Build history of the part. All positions in model axes, mm. Face numbers are marked on the shaded views. A direction names the side the tool comes from. Give positions to 0.01 mm unless a question says otherwise; leave off trailing zeros. Loops run counter-clockwise (first coordinate to the right, second up) from the corner with the lowest first, then second, coordinate; pieces in that order, holes last. Notation, with made-up numbers: M 38,-16 L 83,-16 A18 ccw 83,7 Z; hole C 20,70 d1. An arc over 180 degrees is marked long. Answer as a JSON object with one key per item and string values. Group by question number.
1. Slice it at A-A (y = 13.5). List the corners of the cut face in (x, z).
2. Slice it at B-B (z = 9.5). List the corners of the cut face in (x, y), then the cut area to 3 significant figures.
3. Slice it at C-C (x = -11.5). List the corners of the cut face in (y, z).
4. Mould opens along X. For the marked faces 3, 4 and 5 say: released by +X, released by -X, zero draft, split by the parting line, or undercut.
5. 3-axis set-ups, long thin cutter, end or side, ignore diameter. For the marked faces 1 and 2: which of +Z, -Z, +X, -X, +Y, -Y reach the whole face in a straight line?
6. Drill centre lines: line 1 along X through (y, z) = (9, 12.5); line 2 along X through (y, z) = (8.5, 25); line 3 along Z through (x, y) = (-2, 13). Where is each one in solid material? Low to high. Write a range as [from, to].
from build123d import *

# Parameters (mm, degrees)
F0_W     = 60
F0_H     = 6.8944109904
F1_DEPTH = 38
F3_DEPTH = 25


with BuildPart() as f1:
    # F0 (on Top) → F1 (new body)
    with BuildSketch(Plane.XY):
        with Locations((-5.1953140646, 10.8007821254)):
            Rectangle(F0_W, F0_H)
    extrude(amount=F1_DEPTH)

    # F2 (on face) → F3 (cut)
    with BuildSketch(Plane.XZ.offset(-7.3535766302)):
        with BuildLine():
            ThreePointArc((-5.1953140646, 37), (-13.5847741794, 26.3243358859), (-16.1953140646, 13))
            ThreePointArc((-16.1953140646, 13), (-5.1953140646, 2), (5.8046859354, 13))
            ThreePointArc((5.8046859354, 13), (3.1941460502, 26.3243358859), (-5.1953140646, 37))
        make_face()
    extrude(amount=-F3_DEPTH, mode=Mode.SUBTRACT)


solid = f1.part
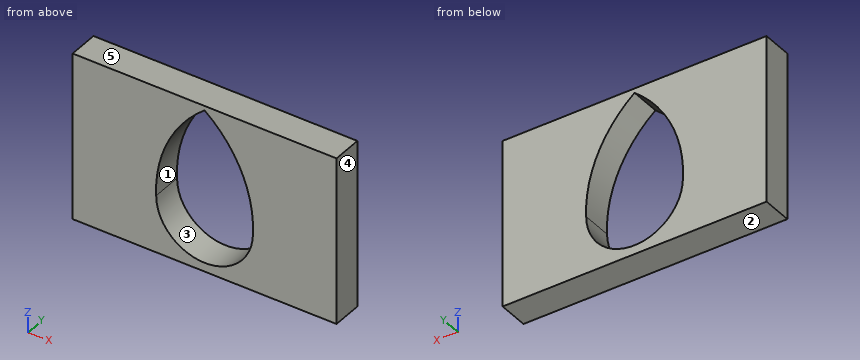
Established:
{
 "1": {"outline": "M -35.2,0 L 24.8,0 L 24.8,38 L -35.2,38 Z; hole M -16.2,13 A11 ccw 5.8,13 A29 ccw -5.2,37 A29 ccw Z"},
 "2": {"outline": "M -35.2,7.35 L -15.62,7.35 L -15.62,14.25 L -35.2,14.25 Z; M 5.23,7.35 L 24.8,7.35 L 24.8,14.25 L 5.23,14.25 Z", "area": "270 mm^2"},
 "3": {"outline": "M 7.35,0 L 14.25,0 L 14.25,3.99 L 7.35,3.99 Z; M 7.35,30.1 L 14.25,30.1 L 14.25,38 L 7.35,38 Z"},
 "4": {"face 3": "undercut", "face 4": "released by +X", "face 5": "zero draft"},
 "5": {"face 1": "+Y, -Y", "face 2": "-Z, +X, -X, +Y, -Y"},
 "6": {"line 1": "x = [-35.2, -16.18], [5.79, 24.8]", "line 2": "x = [-35.2, -14.15], [3.76, 24.8]", "line 3": "z = [0, 2.47], [34.06, 38]"}
}
